```python
from build123d import *


with BuildPart() as part:
    # Szkic1 → Obrót1 (revolve)
    with BuildSketch(Plane.XY, mode=Mode.PRIVATE) as obr_t1_sk:
        with BuildLine():
            Line((-19.02, -51.203493976), (-22.04, -51.203493976))
            Line((-22.04, -51.203493976), (-23.04, -51.203493976))
            Line((-23.04, -51.203493976), (-23.04, -50.203493976))
            Line((-23.04, -50.203493976), (-23.04, 55.796506024))
            Line((-23.04, 55.796506024), (-23.02, 55.796506024))
            ThreePointArc((-23.02, 55.796506024), (-20.191572875, 54.624933149), (-19.02, 51.796506024))
            Line((-19.02, 51.796506024), (-19.02, -41.411476786))
            Line((-19.02, -41.411476786), (0, -41.411476786))
            Line((0, -41.411476786), (0, -50.371476786))
            Line((0, -50.371476786), (-9.51, -50.371476786))
            Line((-9.51, -50.371476786), (-19.02, -51.203493976))
        make_face()
    revolve(obr_t1_sk.sketch.rotate(Axis((0, -51.853493976, 0), (0, 1, 0)), 180), axis=Axis((0, -51.853493976, 0), (0, 1, 0)))


solid = part.part
```
For this review, take the finished solid that the model builds, in its own axes (mm). A direction names the side the tool comes from. Coordinates: 2 decimals unless noted, no trailing zeros. Loops run counter-clockwise (first coordinate to the right, second up) from the corner with the lowest first, then second, coordinate; pieces in that order, holes last.
1. For line 1 (X direction, y = 13, z = 0.5); line 2 (Z direction, x = 0, y = -5.5); line 3 (X direction, y = -40, z = 9), list the stretches that pass through material, from the lowest coordinate up.
2. Add section D-D, the plane y = -43. Give the boundary of the cut face in (x, z), then the cut area to 3 significant figures.
3. Add section C-C, the plane y = 26.5. Give the boundary of the cut face in (x, z), then the cut area to 3 significant figures.
4. Insertion check: P1, Ø1, axis at x = 5.5, y = 5, coming from the -Z side; P2, Ø6, axis at x = -0.5, z = 9, coming from the +Y side; P3, Ø15, axis at x = 2.5, z = -3.5, coming from the -Y side. Each pin has a flat end and moves straight along its axis. Give the tip position at first contact, or say it passes through.
5. Mouldability with a two-part tool opening along X and no side actions: class faces 1 (the flat face through (0, -50.371, 0)), 2 (the flat face through (-3, -51.203, -19)), 3 (the cylindrical face through (21.976, 3.046, -6.921)) as +X half, -X half, draft (parallel to the pull), parting line (faces both ways), or undercut.
6. For faces 4 (the conical face through (9.638, -50.424, -3.035)), 5 (the cylindrical face through (8.78, 4.54, 16.87)), list the 3-axis set-ups (+Z, -Z, +X, -X, +Y, -Y) from which the entire face can be reached by the end or side of a thin tool; tool diameter is ignored.
Result:
1. line 1: x = -23.03 to -19.01, 19.01 to 23.03
1. line 2: z = -23.04 to -19.02, 19.02 to 23.04
1. line 3: x = -21.21 to -16.76, 16.76 to 21.21
2. outline: circle Ø46.08 at (0, 0)
2. area: 1,670 mm2
3. outline: circle Ø46.08 at (0, 0); hole circle Ø38.04 at (0, 0)
3. area: 531 mm2
4. P1: stops at z = -22.49
4. P2: stops at y = -41.41
4. P3: stops at y = -50.57
5. face 1: undercut
5. face 2: draft
5. face 3: parting line
6. face 4: -Y
6. face 5: +Y
